Build history of the part. All positions in model axes, mm. A direction names the side the tool comes from. Coordinates: 2 decimals unless noted, no trailing zeros. Loops run counter-clockwise (first coordinate to the right, second up) from the corner with the lowest first, then second, coordinate; pieces in that order, holes last.
Item 1: Cut at C-C (x = 32). List the corners of the cut face in (y, z), and give its area (3 significant figures).
Item 2: Cut at A-A (y = 64.5). List the corners of the cut face in (x, z), and give its area (3 significant figures).
Item 3: Mould opens along Y. For faces 1 (the face through (5, 65, 150)), 2 (the face through (5, 30, 145)) say: released by +Y, released by -Y, zero draft, split by the parting line, or undercut.
Item 4: 3-axis set-ups, long thin cutter, end or side, ignore diameter. For faces 3 (the face through (85, 75, 140)), 4 (the face through (60, 85, 145)), 5 (the face through (5, 25, 150)), 6 (the face through (45, 45, 126)): which of +Z, -Z, +X, -X, +Y, -Y reach the whole face in a straight line?
Item 5: Flat gauge pins, fed straight in: pin 1 (3 mm diameter, centred on x = 6, y = 17, fed in from +Z); pin 2 (8 mm diameter, centred on x = 68, y = 50.5, fed in from +Z). Where does each tip first touch, or does it go through?
Item 6: Drill centre lines: line 1 along Y through (x, z) = (9, 144); line 2 along Z through (x, y) = (48, 56.5); line 3 along X through (y, z) = (73.5, 131.5). Where is each one in solid material? Low to high.
Item 7: Cut at B-B (x = 6.5). List the corners of the cut face in (y, z).
from build123d import *

# Parameters (mm, degrees)
BOX003_W      = 70
BOX003_H      = 70
BOX003_DEPTH  = 25
BOX001_W      = 10
BOX001_H      = 10
BOX001_DEPTH  = 10
ARRAY_X_COUNT = 5
ARRAY_X_PITCH = 20
ARRAY_Y_COUNT = 5
ARRAY_Y_PITCH = 20
BOX002_W      = 90
BOX002_H      = 90
BOX002_DEPTH  = 10
BOX_W         = 90
BOX_H         = 90
BOX_DEPTH     = 150


with BuildPart() as cub003:
    # Box003 → Box003 (new body)
    with BuildSketch(Plane(origin=(10, 10, 126), x_dir=(1, 0, 0), z_dir=(0, 0, 1))):
        with Locations((35, 35)):
            Rectangle(BOX003_W, BOX003_H)
    extrude(amount=BOX003_DEPTH)


with BuildPart() as array:
    # Box001 → Box001 (new body)
    with BuildSketch(Plane.XY):
        with Locations((5, 5)):
            Rectangle(BOX001_W, BOX001_H)
    extrude(amount=BOX001_DEPTH)

    # Array X: Array ×5


with BuildPart() as array_1:
    add(array.part)
    with Locations(*[(i * ARRAY_X_PITCH, 0, 0) for i in range(1, ARRAY_X_COUNT)]):
        add(array.part)

    # Array Y: Array ×5


with BuildPart() as array_2:
    add(array_1.part)
    with Locations(*[(0, i * ARRAY_Y_PITCH, 0) for i in range(1, ARRAY_Y_COUNT)]):
        add(array_1.part)


with BuildPart() as cut:
    # Box002 → Box002 (new body)
    with BuildSketch(Plane.XY):
        with Locations((45, 45)):
            Rectangle(BOX002_W, BOX002_H)
    extrude(amount=BOX002_DEPTH)

    # Cut: cut Array
    add(array_2.part, mode=Mode.SUBTRACT)


with BuildPart() as cut_1:
    # Cut placement: moved
    add(cut.part.moved(Location((0, 0, 140))))


with BuildPart() as cut002:
    # Box → Box (new body)
    with BuildSketch(Plane.XY):
        with Locations((45, 45)):
            Rectangle(BOX_W, BOX_H)
    extrude(amount=BOX_DEPTH)

    # Cut001: cut Cut
    add(cut_1.part, mode=Mode.SUBTRACT)

    # Cut002: cut Cub003
    add(cub003.part, mode=Mode.SUBTRACT)


solid = cut002.part
Filled sheet:
1. outline: (0, 0) - (90, 0) - (90, 140) - (80, 140) - (80, 126) - (10, 126) - (10, 140) - (0, 140) - close
1. area: 11,600 mm2
2. outline: (0, 0) - (90, 0) - (90, 150) - (80, 150) - (80, 126) - (10, 126) - (10, 150) - (0, 150) - close
2. area: 11,800 mm2
3. face 1: zero draft
3. face 2: undercut
4. face 3: +Z, +X, -X
4. face 4: +Z, +Y, -Y
4. face 5: +Z, +X, -X, +Y, -Y
4. face 6: +Z
5. pin 1: stops at z = 140
5. pin 2: stops at z = 126
6. line 1: y = 0 to 10, 20 to 30, 40 to 50, 60 to 70, 80 to 90
6. line 2: z = 0 to 126
6. line 3: x = 0 to 10, 80 to 90
7. outline: (0, 0) - (90, 0) - (90, 150) - (80, 150) - (80, 140) - (70, 140) - (70, 150) - (60, 150) - (60, 140) - (50, 140) - (50, 150) - (40, 150) - (40, 140) - (30, 140) - (30, 150) - (20, 150) - (20, 140) - (10, 140) - (10, 150) - (0, 150) - close
